Read the model definition and answer for the solid it produces. Units are mm, in the model's axes. A direction names the side the tool comes from. Coordinates: 2 decimals unless noted, no trailing zeros. Write each loop counter-clockwise with the first axis right and the second up, starting at its lowest first coordinate (ties: lowest second). Pieces come first, ordered by that corner, then holes. Notation, with made-up numbers: M 3.25,38 L 8.25,38 A15 ccw 8.25,64 Z; hole C 72.25,14 d10. An arc over 180 degrees is marked long. Write item = value, one per line.
from build123d import *

# Parameters (mm, degrees)
PAD_DEPTH           = 30
SKETCH007_R         = 7.5
PAD006_DEPTH        = 50
SKETCH009_W         = 30
SKETCH009_H         = 40
PAD007_DEPTH        = 108
SKETCH008_R         = 7.349434
POCKET_DEPTH        = 114
HOLE001_D           = 4.2
HOLE001_DEPTH       = 62
HOLE001_CSINK_D     = 11.2
HOLE001_CSINK_ANGLE = 90
SKETCH012_R         = 10
POCKET001_DEPTH     = 42
SKETCH016_W         = 40
SKETCH016_H         = 40
POCKET004_DEPTH     = 10
SKETCH017_R         = 2.1
HOLE002_DEPTH       = 36
POCKET007_DEPTH     = 71


with BuildPart() as part:
    # Sketch → Pad (new body)
    with BuildSketch(Plane.YZ):
        with BuildLine():
            ThreePointArc((100, 0), (-1.8e-05, 100), (-100, -3.5e-05))
            Line((-100, -3.5e-05), (-40, -50))
            Line((-40, -50), (40, -50))
            Line((100, 0), (40, -50))
        make_face()
    extrude(amount=PAD_DEPTH)

    # Sketch007 → Pad006 (join)
    with BuildSketch(Plane.YZ.offset(-15)):
        Circle(SKETCH007_R)
    extrude(amount=PAD006_DEPTH)

    # Sketch009 → Pad007 (join)
    with BuildSketch(Plane.XY):
        with Locations((15, 0)):
            Rectangle(SKETCH009_W, SKETCH009_H)
    extrude(amount=PAD007_DEPTH)

    # Sketch008 → Pocket (cut)
    with BuildSketch(Plane.XY):
        with Locations((15, 0)):
            Circle(SKETCH008_R)
    extrude(amount=POCKET_DEPTH, mode=Mode.SUBTRACT)

    # Hole001
    with Locations(Plane(origin=(0, 0, 0), x_dir=(0, 1, 0), z_dir=(-1, 0, 0))):
        with Locations((0, -45), (0, -30)):
            CounterSinkHole(HOLE001_D / 2, HOLE001_CSINK_D / 2, depth=HOLE001_DEPTH, counter_sink_angle=HOLE001_CSINK_ANGLE)

    # Sketch012 → Pocket001 (cut)
    with BuildSketch(Plane.YZ):
        with Locations((-70, 20)):
            Circle(SKETCH012_R)
        with Locations((70, 20)):
            Circle(SKETCH012_R)
    extrude(amount=POCKET001_DEPTH, mode=Mode.SUBTRACT)

    # Sketch016 → Pocket004 (cut)
    with BuildSketch(Plane.YZ):
        with Locations((-70, 20)):
            Rectangle(SKETCH016_W, SKETCH016_H)
        with Locations((70, 20)):
            Rectangle(SKETCH016_W, SKETCH016_H)
    extrude(amount=POCKET004_DEPTH, mode=Mode.SUBTRACT)

    # Sketch017 → Hole002 (cut)
    with BuildSketch(Plane.YZ):
        with Locations((-82.5, 32.5)):
            Circle(SKETCH017_R)
        with Locations((-57.5, 32.5)):
            Circle(SKETCH017_R)
        with Locations((-82.5, 7.5)):
            Circle(SKETCH017_R)
        with Locations((-57.5, 7.5)):
            Circle(SKETCH017_R)
        with Locations((57.5, 32.5)):
            Circle(SKETCH017_R)
        with Locations((82.5, 32.5)):
            Circle(SKETCH017_R)
        with Locations((57.5, 7.5)):
            Circle(SKETCH017_R)
        with Locations((82.5, 7.5)):
            Circle(SKETCH017_R)
    extrude(amount=HOLE002_DEPTH, mode=Mode.SUBTRACT)

    # Sketch031 → Pocket007 (cut)
    with BuildSketch(Plane.YZ.offset(40)):
        with BuildLine():
            ThreePointArc((2.748601, -1.00041), (0, 2.924999), (-2.748601, -1.00041))
            Line((-2.748601, -1.00041), (2.748601, -1.00041))
        make_face()
    extrude(amount=-POCKET007_DEPTH, mode=Mode.SUBTRACT)


solid = part.part
Item 1: Find section A-A (y = -82.5). Determine the outline of the cut face in (x, z).
Worked answers:
outline = M 0,-14.58 L 30,-14.58 L 30,5.4 L 10,5.4 L 10,0 L 0,0 Z; M 0,40 L 10,40 L 10,34.6 L 30,34.6 L 30,56.51 L 0,56.51 Z; M 10,9.6 L 30,9.6 L 30,30.4 L 10,30.4 Z
Item 2: Consider line 1 along Z through (x, y) = (22, 57); line 2 along Y through (x, z) = (21, 32.5); line 3 along Z through (x, y) = (15.75, -57.5). Determine where each line is inside the solid, lowest interval first. Write a range as from..to.
Worked answers:
line_1 = -35.83..5.46, 9.54..30.46, 34.54..82.16
line_2 = -94.57..-84.6, -80.4..-59.6, -55.4..-4.24, 4.24..55.4, 59.6..80.4, 84.6..94.57
line_3 = -35.42..5.4, 9.6..30.4, 34.6..81.82
Item 3: Which of the six approach directions +Z, -Z, +X, -X, +Y, -Y give full straight-line access (tool end or side, diameter ignored) to faces 1 (the face through (15, -20, 103)), 2 (the face through (5, -50, 20)), 3 (the face through (21.79, -2.81, 53.24)), 4 (the face through (32.465, -7.493, 0.33)), 5 (the face through (10, 0, -1))?
Worked answers:
face_1 = +Z, +X, -X, -Y
face_2 = -X
face_3 = +Z
face_4 = +X
face_5 = +X, -X
Item 4: Flat-ended cylindrical pins translate along their axes: pin 1 (5 mm diameter, centred on y = 82.5, z = 32.5, fed in from +X); pin 2 (4.5 mm diameter, centred on y = 0, z = 0, fed in from -X); pin 3 (10 mm diameter, centred on y = -77.5, z = 78, fed in from -X); pin 4 (5 mm diameter, centred on x = 3.5, z = 21.5, fed in from -Y). Find the tip coordinate at first contact, or state that the pin passes through.
Worked answers:
pin_1 = 30
pin_2 = -15
pin_3 = through
pin_4 = -98.18
Item 5: Find section B-B (x = 15). State how many separate pieces and enclosed holes the cut face has, and give its area (3 significant figures).
Worked answers:
separate_pieces = 1
enclosed_holes = 10
area = 20,700 mm²
Item 6: Find section C-C (z = 20). Determine the outline of the cut face in (x, y), and give its area (3 significant figures).
Worked answers:
outline = M 0,-97.98 L 30,-97.98 L 30,-80 L 10,-80 L 10,-90 L 0,-90 Z; M 0,-50 L 10,-50 L 10,-60 L 30,-60 L 30,60 L 10,60 L 10,50 L 0,50 Z; M 0,90 L 10,90 L 10,80 L 30,80 L 30,97.98 L 0,97.98 Z; hole C 15,0 d14.7
area = 4,110 mm²
Item 7: Find section D-D (z = 53.5). Determine the outline of the cut face in (x, y), and give its area (3 significant figures).
Worked answers:
outline = M 0,-84.49 L 30,-84.49 L 30,84.49 L 0,84.49 Z; hole C 15,0 d14.7
area = 4,900 mm²
Item 8: For a pull along Y with two mould halves and no side action, classify faces 6 (the face through (-15, 0, -2)), 7 (the face through (-7.605, -7.493, 0.33)), 8 (the face through (15, -70, -25)), 9 (the face through (19.86, 58.63, 9.27)) as released by +Y, released by -Y, zero draft, split by the parting line, or undercut.
Worked answers:
face_6 = zero draft
face_7 = split by the parting line
face_8 = released by -Y
face_9 = undercut
